Autodesk Inventor part; units mm, degrees
ref_plane "YZ Plane" through (0, 0, 0) normal (1, 0, 0) x (0, 1, 0)
ref_plane "XZ Plane" through (0, 0, 0) normal (0, 1, 0) x (-1, 0, 0)
ref_plane "XY Plane" through (0, 0, 0) normal (0, 0, 1) x (1, 0, 0)
sketch "Sketch1" plane through (0, 0, 0) normal (0, 0, 1) x (1, 0, 0)
  line L0 (2, 7.5) -> (-2, 7.5)
  line L1 (-5, 4.5) -> (-5, -7.5)
  line L2 (-5, -7.5) -> (5, -7.5)
  line L3 (5, -7.5) -> (5, 4.5)
  line L4 (5, 7.5) -> (-5, -7.5) construction
  line L5 (-5, 7.5) -> (5, -7.5) construction
  arc A0 (-2, 7.5) -> (-5, 4.5) centre (-2, 4.5) ccw
  arc A1 (5, 4.5) -> (2, 7.5) centre (2, 4.5) ccw
  circle A2 centre (0, -4.5) radius 1
  circle A3 centre (0, 0.5) radius 1
  line L6 (-10.3044, 3.5) -> (10.8002, 3.5) construction
  line L7 (-3, -7.5) -> (-3, 3.5)
  line L8 (-3, 3.5) -> (-5, 3.5)
  line L9 (3, -7.5) -> (3, 3.5)
  line L10 (3, 3.5) -> (5, 3.5)
  point P0 (0, 0)
  point P1 (0, 7.5)
  dimension "d0" = 10
  dimension "d1" = 15
  dimension "d2" = 3
  dimension "d3" = 2
  dimension "d4" = 2
  dimension "d5" = 3
  dimension "d6" = 5
  dimension "d9" = 3
  dimension "d10" = 3
  dimension "d11" = 3
extrude "Extrusion1" add sketch "Sketch1" along normal blind 30 contours A1 L3 L10 L9 L2 L7 L8 L1 A0 L0
chamfer "Chamfer1" distance 3.4641 angle 30 1 edges at (3, 3.5, 15) measured on face at (3, -3.8333, 10)
chamfer "Chamfer2" distance 3.4641 angle 30 1 edges at (-3, 3.5, 15) measured on face at (-3, -0.1667, 10)
sketch "Sketch2" plane through (-2, 7.5, 0) normal (0, 1, 0) x (1, 0, 0)
  circle A0 centre (2, -25) radius 1
  circle A1 centre (2, -5) radius 1
  line L0 (4, 0) -> (0, 0)
  line L1 (4, -30) -> (0, -30)
  point P0 (2, 0)
  point P1 (2, 0)
  point P2 (2, 0)
  dimension "d19" = 2
  dimension "d20" = 2
  dimension "d21" = 5
  dimension "d22" = 5
extrude "Extrusion2" cut sketch "Sketch2" against normal blind 3
sketch "Sketch3" plane through (0, 0, 30) normal (0, 0, 1) x (1, 0, 0)
  line L0 (-3, -7.5) -> (3, -7.5)
  line L1 (3, -7.5) -> (7.5, -7.5) construction
  line L2 (7.5, -7.5) -> (7.5, 4.5) construction
  line L3 (7.5, 4.5) -> (5, 4.5) construction
  line L4 (3, 4.5) -> (3, -7.5) construction
  line L5 (7.5, 4.5) -> (3, -0.8629)
  line L6 (7.5, 4.5) -> (13.864, 4.5) construction
  line L7 (7.5, 4.5) -> (5, 4.5)
  line L8 (5, 3.5) -> (3, 0.0359)
  line L9 (5, 3.5) -> (5, 4.5)
  line L10 (3, -7.5) -> (3, 0.0359)
  point P0 (0, 0)
  dimension "d25" = 4.5
  dimension "d26" = 12
  dimension "d27" = 130
extrude "Extrusion3" add sketch "Sketch3" against normal up to surface (30 mm away)
mirror "Mirror2" about plane through (0, 0, 0) normal (1, 0, 0) of "Extrusion3"
properties part number "Foot_V1"
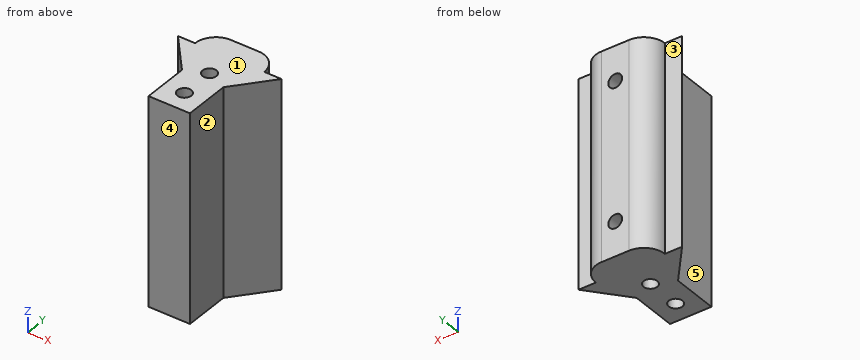
For this review, take the finished solid that the model builds, in its own axes (mm). Face numbers are marked on the shaded views. A direction names the side the tool comes from. Give positions to 0.01 mm unless a question says otherwise; leave off trailing zeros. Loops run counter-clockwise (first coordinate to the right, second up) from the corner with the lowest first, then second, coordinate; pieces in that order, holes last. Notation, with made-up numbers: M 7,71 L 18,71 A16 ccw 18,77 Z; hole C -23,63.5 d6. An arc over 180 degrees is marked long. One line per item, written item: value. Start each with the question number.
Q1. For L1, parallel to Y at x = 0, z = 18; L2, parallel to Z at x = 0, y = 5.65; L3, parallel to X at y = -3.25, z = 26, list the stretches that pass through material, from the lowest coordinate up.
Q2. Machinability: for the marked faces 1 and 2, which of the approach directions +Z, -Z, +X, -X, +Y, -Y give a long, thin tool a straight path to every point of the face, cutting with its end or side? Answer none if there is none.
Q3. Draft analysis for pull direction Y (two halves, no side actions). For the marked faces 3, 4 and 5, state which applies: released by +Y, released by -Y, zero draft, split by the parting line, or undercut.
Q4. Add section A-A (x = 0). Give the boundary of the cut face in (y, z), and give its area (3 significant figures).
Q5. Add section D-D (y = -2.5). Give the boundary of the cut face in (x, z).
Q6. Add section B-B (y = -4.5). Give the boundary of the cut face in (x, z), and give its area (3 significant figures).
Q7. Clearance check with flat-ended pins moving along their axes: pin 1 Ø8 at (y, z) = (-4, 13) entering from -X; pin 2 Ø1.2 at (x, z) = (-6, 12.5) entering from +Y; pin 3 Ø4 at (x, z) = (5.5, 12.5) entering from +Y. State where each tip first meets the part, or that it passes through.
Q8. Add section C-C (z = 5). Give the boundary of the cut face in (x, y), and give its area (3 significant figures).
Reply:
1. L1: -7.5 to -5.5, -3.5 to -0.5, 1.5 to 7.5
1. L2: 0 to 4, 6 to 24, 26 to 30
1. L3: -3 to 3
2. face 1: +Z, +X, -X, +Y, -Y
2. face 2: +Z, -Z, +X, -Y
3. face 3: released by +Y
3. face 4: released by -Y
3. face 5: zero draft
4. outline: M -7.5,0 L -5.5,0 L -5.5,30 L -7.5,30 Z; M -3.5,0 L -0.5,0 L -0.5,30 L -3.5,30 Z; M 1.5,0 L 7.5,0 L 7.5,4 L 4.5,4 L 4.5,6 L 7.5,6 L 7.5,24 L 4.5,24 L 4.5,26 L 7.5,26 L 7.5,30 L 1.5,30 Z
4. area: 318 mm²
5. outline: M -3,0 L 3,0 L 3,30 L -3,30 Z
6. outline: M -3,0 L -1,0 L -1,30 L -3,30 Z; M 1,0 L 3,0 L 3,30 L 1,30 Z
6. area: 120 mm²
7. pin 1: x = -3.72
7. pin 2: y = 4.5
7. pin 3: y = 7.1
8. outline: M -7.5,4.5 L -3,-0.86 L -3,-7.5 L 3,-7.5 L 3,-0.86 L 7.5,4.5 L 5,4.5 A3 ccw 2,7.5 L 1,7.5 L 1,4.5 L -1,4.5 L -1,7.5 L -2,7.5 A3 ccw -5,4.5 Z; hole C 0,-4.5 d2; hole C 0,0.5 d2
8. area: 110 mm²
